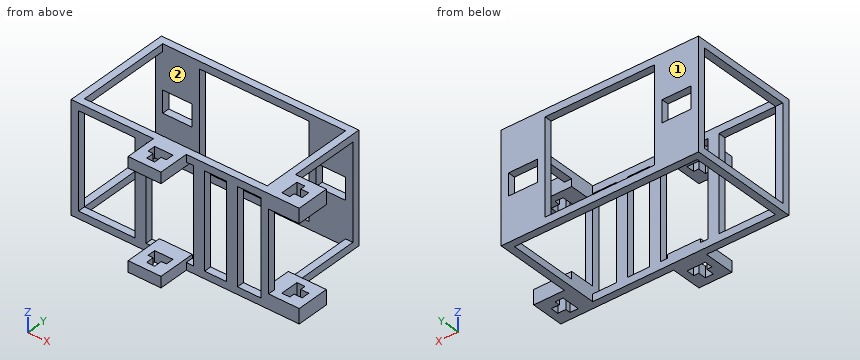
```python
from build123d import *

# Parameters (mm, degrees)
SKETCH1_W           = 54
SKETCH1_H           = 30
SKETCH1_W_2         = 50
SKETCH1_H_2         = 26
BOSS_EXTRUDE1_DEPTH = 2
SKETCH2_W           = 2
SKETCH2_H           = 2
BOSS_EXTRUDE2_DEPTH = 28
SKETCH3_W           = 2
SKETCH3_H           = 9
BOSS_EXTRUDE3_DEPTH = 4
BOSS_EXTRUDE4_DEPTH = 3
SKETCH6_W           = 2
SKETCH6_H           = 2
BOSS_EXTRUDE5_DEPTH = 2
SKETCH10_W          = 3
SKETCH10_H          = 26
BOSS_EXTRUDE7_DEPTH = 2
SKETCH11_W          = 2
SKETCH11_H          = 6
BOSS_EXTRUDE9_DEPTH = 2


with BuildPart() as part:
    # Sketch1 → Boss-Extrude1 (new body)
    with BuildSketch(Plane(origin=(0, 0, 0), x_dir=(1, 0, 0), z_dir=(0, 1, 0))):
        Rectangle(SKETCH1_W, SKETCH1_H)
        Rectangle(SKETCH1_W_2, SKETCH1_H_2, mode=Mode.SUBTRACT)
    extrude(amount=BOSS_EXTRUDE1_DEPTH)

    # Sketch2 → Boss-Extrude2 (add)
    with BuildSketch(Plane(origin=(0, 0, 0), x_dir=(1, 0, 0), z_dir=(0, 1, 0))):
        with Locations((26, 14)):
            Rectangle(SKETCH2_W, SKETCH2_H)
        with Locations((26, -14)):
            Rectangle(SKETCH2_W, SKETCH2_H)
        with Locations((-26, -14)):
            Rectangle(SKETCH2_W, SKETCH2_H)
        with Locations((-26, 14)):
            Rectangle(SKETCH2_W, SKETCH2_H)
    extrude(amount=BOSS_EXTRUDE2_DEPTH)

    # Sketch3 → Boss-Extrude3 (add)
    with BuildSketch(Plane.XY.offset(15)):
        Polygon((27, 9), (27, 4.5), (29, 4.5), (29, 7), (31.2, 7), (31.2, 5.6), (33.4, 5.6), (33.4, 4.5), (35.4, 4.5), (35.4, 9), align=None)
        Polygon((27, 4.5), (27, 0), (35.4, 0), (35.4, 4.5), (33.4, 4.5), (33.4, 3.4), (31.2, 3.4), (31.2, 2), (29, 2), (29, 4.5), align=None)
        with Locations((26, 4.5)):
            Rectangle(SKETCH3_W, SKETCH3_H)
    boss_extrude3 = extrude(amount=-BOSS_EXTRUDE3_DEPTH)

    # Mirror1: Boss-Extrude3 across plane
    add(boss_extrude3.mirror(Plane.XY))

    # Sketch4 → Boss-Extrude4 (add)
    with BuildSketch(Plane.XY.offset(15)):
        Polygon((-4.5, 0), (0, 0), (4.5, 0), (4.5, 2), (-4.5, 2), align=None)
        Polygon((4.5, 0), (0, 0), (-4.5, 0), (-4.5, -8.4), (0, -8.4), (4.5, -8.4), align=None)
        Polygon((1.1, -6.4), (0, -6.4), (-1.1, -6.4), (-1.1, -4.2), (-2.5, -4.2), (-2.5, -2), (2.5, -2), (2.5, -4.2), (1.1, -4.2), align=None, mode=Mode.SUBTRACT)
    boss_extrude4 = extrude(amount=-BOSS_EXTRUDE4_DEPTH)

    # Mirror2: Boss-Extrude4 across plane
    add(boss_extrude4.mirror(Plane.XY))

    # Sketch6 → Boss-Extrude5 (add)
    with BuildSketch(Plane(origin=(0, 28, 0), x_dir=(1, 0, 0), z_dir=(0, 1, 0))):
        with Locations((26, -14)):
            Rectangle(SKETCH6_W, SKETCH6_H)
        Polygon((-27, -15), (25, -15), (25, -13), (27, -13), (27, 15), (-27, 15), align=None)
        Polygon((25, 6), (25, -13), (-25, -13), (-25, -9), (-25, 6), (-25, 9), (-25, 13), (25, 13), (25, 9), align=None, mode=Mode.SUBTRACT)
    extrude(amount=BOSS_EXTRUDE5_DEPTH)

    # Sketch10 → Boss-Extrude7 (add)
    with BuildSketch(Plane(origin=(0, 2, 0), x_dir=(1, 0, 0), z_dir=(0, 1, 0))):
        with Locations((8, 0)):
            Rectangle(SKETCH10_W, SKETCH10_H)
        with Locations((-8, 0)):
            Rectangle(SKETCH10_W, SKETCH10_H)
        with Locations((17, 0)):
            Rectangle(SKETCH10_W, SKETCH10_H)
    extrude(amount=-BOSS_EXTRUDE7_DEPTH)

    # Sketch11 → Boss-Extrude9 (add)
    with BuildSketch(Plane(origin=(0, 30, 0), x_dir=(1, 0, 0), z_dir=(0, 1, 0))):
        Polygon((15, -3), (15, -13), (25, -13), (25, -3), (17, -3), align=None)
        with Locations((16, 0)):
            Rectangle(SKETCH11_W, SKETCH11_H)
        Polygon((15, 13), (15, 3), (17, 3), (25, 3), (25, 13), align=None)
        Polygon((-17, 3), (-15, 3), (-15, 13), (-25, 13), (-25, 3), align=None)
        Polygon((-25, -3), (-25, -13), (-15, -13), (-15, -3), (-17, -3), align=None)
        with Locations((-16, 0)):
            Rectangle(SKETCH11_W, SKETCH11_H)
    extrude(amount=-BOSS_EXTRUDE9_DEPTH)


solid = part.part
```
Verification items for the finished model (mm, model axes). Face numbers are marked on the shaded views. Give positions to 0.01 mm unless a question says otherwise; leave off trailing zeros. Order: outer loops, then holes, each group sorted by start corner. A loop starts at its lowest first (then second) coordinate and runs counter-clockwise, first axis right, second up. Notation, with made-up numbers: (68.5, 23) -> (105.5, 23) arc R32 cw to (105.5, 62) -> close; hole circle Ø4 at (57.25, 24.5). An arc over 180 degrees is marked (long way). One line per item, written item: value.
(1) Sectioned sample at D-D on y = 17.5. Record the cut outline in (x, z), then the cut area to 3 significant figures.
Final values:
outline: (-27, -15) -> (-25, -15) -> (-25, -13) -> (-27, -13) -> close; (-27, 13) -> (-25, 13) -> (-25, 15) -> (-27, 15) -> close; (25, -15) -> (27, -15) -> (27, -13) -> (25, -13) -> close; (25, 13) -> (27, 13) -> (27, 15) -> (25, 15) -> close
area: 16.0 mm^2
(2) Gauge pin test, flat ends, axial feed: pin 1 (0.7 mm diameter, centred on y = -5.5, z = -14, fed in from +X); pin 2 (4 mm diameter, centred on x = -8, z = -1.5, fed in from +Y); pin 3 (1 mm diameter, centred on x = -13.5, z = 5, fed in from -Y); pin 4 (17 mm diameter, centred on y = 24.5, z = -1, fed in from +X). Record the tip position at first contact, or that the pin passes through.
Final values:
pin 1: x = 4.5
pin 2: y = 2
pin 3: through
pin 4: x = 27
(3) Sectioned sample at B-B on y = 4.5. Record the cut outline in (x, z), then the cut area to 3 significant figures.
Final values:
outline: (-27, -15) -> (-25, -15) -> (-25, -13) -> (-27, -13) -> close; (-27, 13) -> (-25, 13) -> (-25, 15) -> (-27, 15) -> close; (25, -15) -> (29, -15) -> (29, -11) -> (25, -11) -> close; (25, 11) -> (29, 11) -> (29, 15) -> (25, 15) -> close; (33.4, -15) -> (35.4, -15) -> (35.4, -11) -> (33.4, -11) -> close; (33.4, 11) -> (35.4, 11) -> (35.4, 15) -> (33.4, 15) -> close
area: 56.0 mm^2
(4) Sectioned sample at A-A on x = -21. Record the cut outline in (y, z).
Final values:
outline: (0, -15) -> (2, -15) -> (2, -13) -> (0, -13) -> close; (0, 13) -> (2, 13) -> (2, 15) -> (0, 15) -> close; (28, -15) -> (30, -15) -> (30, -3) -> (28, -3) -> close; (28, 3) -> (30, 3) -> (30, 15) -> (28, 15) -> close
(5) Scan lines: line 1 along X through (y, z) = (3, 12.25); line 2 along Z through (x, y) = (-20.5, 0.5); line 3 along Y through (x, z) = (5.5, 13.5). Record each from-to range of solid material in increasing order. Write a range as [from, to].
Final values:
line 1: [25, 29], [31.2, 35.4]
line 2: [-15, -13], [13, 15]
line 3: [0, 2], [28, 30]
(6) Sectioned sample at C-C on z = -8. Record the cut outline in (x, y), then the cut area to 3 significant figures.
Final values:
outline: (-27, 0) -> (-25, 0) -> (-25, 2) -> (-27, 2) -> close; (-27, 28) -> (-15, 28) -> (-15, 30) -> (-27, 30) -> close; (-9.5, 0) -> (-6.5, 0) -> (-6.5, 2) -> (-9.5, 2) -> close; (6.5, 0) -> (9.5, 0) -> (9.5, 2) -> (6.5, 2) -> close; (15, 28) -> (27, 28) -> (27, 30) -> (15, 30) -> close; (15.5, 0) -> (18.5, 0) -> (18.5, 2) -> (15.5, 2) -> close; (25, 0) -> (27, 0) -> (27, 2) -> (25, 2) -> close
area: 74.0 mm^2
(7) Draft check along X on the marked faces 1 and 2. Enter one of: pulls with the +X half, pulls with the -X half, needs draft (parallel to the pull), parting line crosses it, or undercut.
Final values:
face 1: needs draft
face 2: undercut
